Here's how the part is built. I have some questions about the finished solid (model axes, mm). A direction names the side the tool comes from. Round coordinates to 2 decimals unless told otherwise and drop trailing zeros. Order: outer loops, then holes, each group sorted by start corner. A loop starts at its lowest first (then second) coordinate and runs counter-clockwise, first axis right, second up. Notation, with made-up numbers: (-32.5, 32.25) -> (24.5, 32.25) arc R29 cw to (24.5, 62.25) -> close; hole circle Ø9 at (61, -26.5). An arc over 180 degrees is marked (long way). One line per item, written item: value.
```python
from build123d import *

# Parameters (mm, degrees)
F0_W     = 96.488521
F0_H     = 76.829273
F1_DEPTH = 25
F2_R     = 24.383557
F3_T     = -2


with BuildPart() as f1:
    # F0 (on Top) → F1 (new body)
    with BuildSketch(Plane.XY):
        with Locations((-1.468796, -3.276543)):
            Rectangle(F0_W, F0_H)
    extrude(amount=F1_DEPTH)

    # F2
    f2_edges = [f1.edges().sort_by_distance(p)[0] for p in [
        (46.775464, -41.69118, 12.5),
        (46.775464, 35.138093, 12.5),
        (-49.713057, 35.138093, 12.5),
        (-49.713057, -41.69118, 12.5),
    ]]
    fillet(f2_edges, radius=F2_R)

    # F3
    f3_openings = [f1.faces().sort_by_distance(p)[0] for p in [
        (-1.468796, -3.276544, 25),
    ]]
    offset(amount=F3_T, openings=f3_openings)


solid = f1.part
```
Q1. I need wall thicknesses on line 1 along X through (y, z) = (11, 12.75); line 2 along Y through (x, z) = (4, 18.5); line 3 along Z through (x, y) = (-10.5, -1). Which ranges of each line are inside material? Lowest first, please.
Answers:
line 1: -49.71 to -47.71, 44.77 to 46.77
line 2: -41.69 to -39.69, 33.14 to 35.14
line 3: 0 to 2
Q2. I want a section at A-A on z = 6.5. Write out the boundary of the cut face in (x, y), then the cut area to 3 significant figures.
Answers:
outline: (-49.71, -17.31) arc R24.38 ccw to (-25.33, -41.69) -> (22.39, -41.69) arc R24.38 ccw to (46.78, -17.31) -> (46.78, 10.75) arc R24.38 ccw to (22.39, 35.14) -> (-25.33, 35.14) arc R24.38 ccw to (-49.71, 10.75) -> close; hole (-47.71, -17.31) arc R22.38 ccw to (-25.33, -39.69) -> (22.39, -39.69) arc R22.38 ccw to (44.78, -17.31) -> (44.78, 10.75) arc R22.38 ccw to (22.39, 33.14) -> (-25.33, 33.14) arc R22.38 ccw to (-47.71, 10.75) -> close
area: 597 mm2
Q3. I want a section at B-B on y = 1.5. Write out the boundary of the cut face in (x, z), then the cut area to 3 significant figures.
Answers:
outline: (-49.71, 0) -> (46.78, 0) -> (46.78, 25) -> (44.78, 25) -> (44.78, 2) -> (-47.71, 2) -> (-47.71, 25) -> (-49.71, 25) -> close
area: 285 mm2
Q4. If we mould it in two halves opening along X, with no side actions, what happens to faces 1 (the face through (-2, 33.138, 13)), 2 (the face through (-49.713, -3, 12)), 3 (the face through (-41.33, -32.96, 13.66)), 4 (the face through (39.44, -34.74, 12.68))? For each: pulls with the +X half, pulls with the -X half, needs draft (parallel to the pull), parting line crosses it, or undercut.
Answers:
face 1: undercut
face 2: pulls with the -X half
face 3: undercut
face 4: pulls with the +X half
Q5. For P1, Ø3, axis at x = 28, z = 21, coming from the +Y side; P2, Ø6, axis at y = -21, z = 11.5, coming from the -X side; P3, Ø1, axis at x = -6, y = -9, coming from the +Z side, each with a flat end and sliding along its axis, tell me the tip position at first contact or that it passes through.
Answers:
P1: y = 34.79
P2: x = -49.7
P3: z = 2
Q6. Which directions (+Z, -Z, +X, -X, +Y, -Y) give clear straight access to the entire face, cutting with the end or side of a thin tool? Please do faces 5 (the face through (-2, 35.138, 12)), 6 (the face through (-41.33, 26.41, 13.66)).
Answers:
face 5: +Z, -Z, +X, -X, +Y
face 6: +Z
Q7. I want a section at C-C on x = -9.5. Write out the boundary of the cut face in (y, z).
Answers:
outline: (-41.69, 0) -> (35.14, 0) -> (35.14, 25) -> (33.14, 25) -> (33.14, 2) -> (-39.69, 2) -> (-39.69, 25) -> (-41.69, 25) -> close
